The model under review builds one solid part; all positions refer to its coordinate system, in mm. A direction names the side the tool comes from. Give positions to 0.01 mm unless a question says otherwise; leave off trailing zeros. Order: outer loops, then holes, each group sorted by start corner. A loop starts at its lowest first (then second) coordinate and runs counter-clockwise, first axis right, second up. Notation, with made-up numbers: (60.25, 6.5) - (113.25, 6.5) arc R18 cw to (113.25, 15.5) - close; hole circle Ø6 at (-14.5, -14). An arc over 180 degrees is marked (long way). Use CSV: the item, a comma, the result in double quotes. Start each with the question number.
1. Machinability: for faces 5 (the cylindrical face through (-8.5, 1.5, 46.5)), 6 (the flat face through (-41, 1, 40)), 7 (the cylindrical face through (-16.324, 1.479, 35.542)), which of the approach directions +Z, -Z, +X, -X, +Y, -Y give a long, thin tool a straight path to every point of the face, cutting with its end or side? Answer none if there is none.
2. For pin 1 (1.5 mm diameter, centred on x = -7.5, y = 1.5, fed in from -Z); pin 2 (1.5 mm diameter, centred on y = 2.5, z = 37.5, fed in from +X), all flat-tipped, find the tip position at first contact; note any pin that passes through.
3. Take a section at D-D, the plane x = -24. State the section outline as (y, z) points, then the cut area to 3 significant figures.
4. To check wall thickness, follow line 1 (Z direction, x = -56, y = 2.05); line 2 (X direction, y = 1.45, z = 35.75); line 3 (Z direction, x = -24, y = 2.3). State the ranges of each line that lie inside material, in increasing order. Write a range as [from, to].
5. Take a section at A-A, the plane x = -56. State the section outline as (y, z) points.
6. Draft analysis for pull direction Z (two halves, no side actions). For faces 1 (the flat face through (-16.326, 1.479, 46.91)), 2 (the cylindrical face through (38.49, 1.48, 47.48)), 3 (the cylindrical face through (-55.26, 1.48, 38.42)), 4 (the cylindrical face through (-23.26, 1.48, 38.42)), state which applies: released by +Z, released by -Z, zero draft, split by the parting line, or undercut.
7. Take a section at B-B, the plane z = 37. State the section outline as (x, y) points, then the cut area to 3 significant figures.
8. Take a section at C-C, the plane x = 20.5. State the section outline as (y, z) points, then the cut area to 3 significant figures.
```python
from build123d import *

# Parameters (mm, degrees)
SKETCH_1_R          = 1.6
SKETCH_1_R_2        = 1
SKETCH_1_W          = 24
SKETCH_1_H          = 13
EXTRUDE_1_DEPTH     = 3
SKETCH_2_R          = 1.6
SKETCH_2_W          = 24
SKETCH_2_H          = 10
EXTRUDE_2_DEPTH     = 9
SKETCH_3_R          = 6
CUT_EXTRUDE_1_DEPTH = 20
SKETCH_4_R          = 4
CUT_EXTRUDE_2_DEPTH = 72.704206567
SKETCH_6_R          = 5.6
CUT_EXTRUDE_3_DEPTH = 5
SKETCH_7_R          = 5.6
CUT_EXTRUDE_4_DEPTH = 6
FILLET_5_R          = 5
FILLET_6_R          = 5
CUT_EXTRUDE1_DEPTH  = 13.0000001
FILLET1_R           = 2


with BuildPart() as part:
    # Эскиз1 → Бобышка-Вытянуть1 (new body)
    with BuildSketch(Plane(origin=(0, 0, 0), x_dir=(1, 0, 0), z_dir=(0, 1, 0))):
        with BuildLine():
            Line((-59.846473334, -34), (-49.887758312, 18))
            Line((-49.887758312, 18), (36.612736258, 18))
            Line((36.612736258, 18), (75.112241688, 5.920216985))
            Line((75.112241688, 5.920216985), (75.112241688, -16.079783015))
            Line((75.112241688, -16.079783015), (41.245672077, -52.430849732))
            ThreePointArc((41.245672077, -52.430849732), (39.914841322, -53.372078747), (38.318998701, -53.704206567))
            Line((38.318998701, -53.704206567), (-9.799827382, -53.704206567))
            ThreePointArc((-9.799827382, -53.704206567), (-12.412320205, -52.967407389), (-14.254860003, -50.974159066))
            Line((-14.254860003, -50.974159066), (-19.846473334, -40))
            Line((-19.846473334, -40), (-59.846473334, -40))
            Line((-59.846473334, -40), (-59.846473334, -34))
        make_face()
        with Locations((-8, 14)):
            Circle(SKETCH_1_R, mode=Mode.SUBTRACT)
        with Locations((8, 14)):
            Circle(SKETCH_1_R, mode=Mode.SUBTRACT)
        with Locations((-8, -16)):
            Circle(SKETCH_1_R, mode=Mode.SUBTRACT)
        with Locations((8, -16)):
            Circle(SKETCH_1_R, mode=Mode.SUBTRACT)
        with Locations((-47, 14)):
            Circle(SKETCH_1_R, mode=Mode.SUBTRACT)
        with Locations((70, 2)):
            Circle(SKETCH_1_R, mode=Mode.SUBTRACT)
        with Locations((50, 2)):
            Circle(SKETCH_1_R, mode=Mode.SUBTRACT)
        with Locations((18, 14)):
            Circle(SKETCH_1_R, mode=Mode.SUBTRACT)
        with Locations((-47, -16)):
            Circle(SKETCH_1_R, mode=Mode.SUBTRACT)
        with Locations((-56, -37)):
            Circle(SKETCH_1_R, mode=Mode.SUBTRACT)
        with Locations((-24, -37)):
            Circle(SKETCH_1_R, mode=Mode.SUBTRACT)
        with Locations((50, -16)):
            Circle(SKETCH_1_R, mode=Mode.SUBTRACT)
        with Locations((70, -16)):
            Circle(SKETCH_1_R, mode=Mode.SUBTRACT)
        with Locations((-9, -50.704206567)):
            Circle(SKETCH_1_R, mode=Mode.SUBTRACT)
        with Locations((36, -50.704206567)):
            Circle(SKETCH_1_R, mode=Mode.SUBTRACT)
        with Locations((60, -7)):
            Circle(SKETCH_1_R, mode=Mode.SUBTRACT)
        with Locations((-42, -8)):
            Circle(SKETCH_1_R_2, mode=Mode.SUBTRACT)
        with Locations((-14, -8)):
            Circle(SKETCH_1_R_2, mode=Mode.SUBTRACT)
        with Locations((-42, 8)):
            Circle(SKETCH_1_R_2, mode=Mode.SUBTRACT)
        with Locations((-14, 8)):
            Circle(SKETCH_1_R_2, mode=Mode.SUBTRACT)
        with Locations((14, 0)):
            Circle(SKETCH_1_R_2, mode=Mode.SUBTRACT)
        with Locations((42, 0)):
            Circle(SKETCH_1_R_2, mode=Mode.SUBTRACT)
        with Locations((28, 0)):
            Rectangle(SKETCH_1_W, SKETCH_1_H, mode=Mode.SUBTRACT)
        with Locations((-28, 8)):
            Rectangle(SKETCH_1_W, SKETCH_1_H, mode=Mode.SUBTRACT)
        with Locations((-28, -8)):
            Rectangle(SKETCH_1_W, SKETCH_1_H, mode=Mode.SUBTRACT)
        with BuildLine():
            Line((-47.677053254, -24.900709984), (-49.000145857, -34))
            Line((-49.000145857, -34), (-22.297676486, -34))
            Line((-22.297676486, -34), (-19.846473334, -34))
            ThreePointArc((-19.846473334, -34), (-16.425778662, -35.467187694), (-13.988679802, -38.280431537))
            Line((-13.988679802, -38.280431537), (-11.413907263, -43.333707171))
            ThreePointArc((-11.413907263, -43.333707171), (-8.465843587, -46.522904488), (-4.28585507, -47.701783173))
            Line((-4.28585507, -47.701783173), (34.165827616, -47.701783173))
            ThreePointArc((34.165827616, -47.701783173), (37.877016972, -46.788889321), (40.741225842, -44.258551563))
            Line((40.741225842, -44.258551563), (51.02606102, -29.417576293))
            ThreePointArc((51.02606102, -29.417576293), (51.409841961, -23.216607983), (46.09451235, -20))
            Line((46.09451235, -20), (-41.778616049, -20))
            ThreePointArc((-41.778616049, -20), (-45.612951708, -21.385038456), (-47.677053254, -24.900709984))
        make_face(mode=Mode.SUBTRACT)
    extrude(amount=EXTRUDE_1_DEPTH)

    # Эскиз2 → Бобышка-Вытянуть2 (add)
    with BuildSketch(Plane(origin=(0, 0, 0), x_dir=(1, 0, 0), z_dir=(0, 1, 0))):
        Polygon((46.101706289, 15.022696844), (46.09451235, -20), (71.459960933, -20), (75.112241688, -16.079783015), (75.112241688, 5.920216985), align=None)
        with Locations((50, 2)):
            Circle(SKETCH_2_R, mode=Mode.SUBTRACT)
        with Locations((70, 2)):
            Circle(SKETCH_2_R, mode=Mode.SUBTRACT)
        with Locations((70, -16)):
            Circle(SKETCH_2_R, mode=Mode.SUBTRACT)
        with Locations((50, -16)):
            Circle(SKETCH_2_R, mode=Mode.SUBTRACT)
        with Locations((60, -7)):
            Circle(SKETCH_2_R, mode=Mode.SUBTRACT)
        with Locations((0, 13)):
            Rectangle(SKETCH_2_W, SKETCH_2_H)
        with Locations((-8, 14)):
            Circle(SKETCH_2_R, mode=Mode.SUBTRACT)
        with Locations((8, 14)):
            Circle(SKETCH_2_R, mode=Mode.SUBTRACT)
        with Locations((0, -14.961092538)):
            Rectangle(SKETCH_2_W, SKETCH_2_H)
        with Locations((-8, -16)):
            Circle(SKETCH_2_R, mode=Mode.SUBTRACT)
        with Locations((8, -16)):
            Circle(SKETCH_2_R, mode=Mode.SUBTRACT)
    extrude(amount=-EXTRUDE_2_DEPTH)

    # Эскиз3 → Вырез-Вытянуть1 (cut)
    with BuildSketch(Plane(origin=(75.112241688, 0, 0), x_dir=(0, 0, -1), z_dir=(1, 0, 0))):
        with Locations((-7.384625177, -9)):
            Circle(SKETCH_3_R)
    extrude(amount=-CUT_EXTRUDE_1_DEPTH, mode=Mode.SUBTRACT)

    # Эскиз4 → Вырез-Вытянуть2 (cut, through all)
    with BuildSketch(Plane(origin=(0, 0, -18), x_dir=(-1, 0, 0), z_dir=(0, 0, -1))):
        with Locations((0, -9)):
            Circle(SKETCH_4_R)
    extrude(amount=-CUT_EXTRUDE_2_DEPTH, mode=Mode.SUBTRACT)

    # Эскиз6 → Вырез-Вытянуть3 (cut)
    with BuildSketch(Plane(origin=(0, 0, -18), x_dir=(-1, 0, 0), z_dir=(0, 0, -1))):
        with Locations((0, -9)):
            Circle(SKETCH_6_R)
    extrude(amount=-CUT_EXTRUDE_3_DEPTH, mode=Mode.SUBTRACT)

    # Эскиз7 → Вырез-Вытянуть4 (cut)
    with BuildSketch(Plane.XY.offset(19.961092538)):
        with Locations((0, -9)):
            Circle(SKETCH_7_R)
    extrude(amount=-CUT_EXTRUDE_4_DEPTH, mode=Mode.SUBTRACT)

    # Скругление5
    fillet_5_edges = [part.edges().sort_by_distance(p)[0] for p in [
        (-49.887758312, 1.5, -18),
    ]]
    fillet(fillet_5_edges, radius=FILLET_5_R)

    # Скругление6
    fillet_6_edges = [part.edges().sort_by_distance(p)[0] for p in [
        (-19.846473334, 1.5, 40),
    ]]
    fillet(fillet_6_edges, radius=FILLET_6_R)

    # Sketch1 → Cut-Extrude1 (cut, through all)
    with BuildSketch(Plane(origin=(0, 3, 0), x_dir=(1, 0, 0), z_dir=(0, 1, 0))):
        with BuildLine():
            Line((-59.846473334, -34), (-49.000145857, -34))
            Line((-49.000145857, -34), (39.05274243, -34.20975492))
            Line((39.05274243, -34.20975492), (39.05274243, -46.035665363))
            Line((39.05274243, -46.035665363), (39.914841322, -53.372078747))
            ThreePointArc((39.914841322, -53.372078747), (27.574901916, 149.639179971), (-59.846473334, -34))
        make_face()
    extrude(amount=-CUT_EXTRUDE1_DEPTH, mode=Mode.SUBTRACT)

    # Fillet1
    fillet1_edges = [part.edges().sort_by_distance(p)[0] for p in [
        (39.914841322, 1.5, 53.372078747),
        (39.05274243, 1.5, 46.035665363),
    ]]
    fillet(fillet1_edges, radius=FILLET1_R)


solid = part.part
```
Determined:
1,face 5,"-Z, +Y, -Y"
1,face 6,"+Z, -X, +Y, -Y"
1,face 7,"-Z, +X, +Y, -Y"
2,pin 1,"stops at z = 46.65"
2,pin 2,"stops at x = -14"
3,outline,"(0, 34.06) - (3, 34.06) - (3, 35.4) - (0, 35.4) - close; (0, 38.6) - (3, 38.6) - (3, 40) - (0, 40) - close"
3,area,"8.22 mm²"
4,line 1,"z = [34, 35.4], [38.6, 40]"
4,line 2,"x = [-59.85, -57], [-55, -25], [-23, -16.06]"
4,line 3,"z = [34.06, 35.4], [38.6, 40]"
5,outline,"(0, 34) - (3, 34) - (3, 35.4) - (0, 35.4) - close; (0, 38.6) - (3, 38.6) - (3, 40) - (0, 40) - close"
6,face 1,"released by +Z"
6,face 2,"released by -Z"
6,face 3,"undercut"
6,face 4,"undercut"
7,outline,"(-59.85, 0) - (-57.6, 0) - (-57.6, 3) - (-59.85, 3) - close; (-54.4, 0) - (-25.6, 0) - (-25.6, 3) - (-54.4, 3) - close; (-22.4, 0) - (-14.83, 0) - (-14.83, 3) - (-22.4, 3) - close"
7,area,"116 mm²"
8,outline,"(0, 47.7) - (3, 47.7) - (3, 53.7) - (0, 53.7) - close"
8,area,"18.0 mm²"
